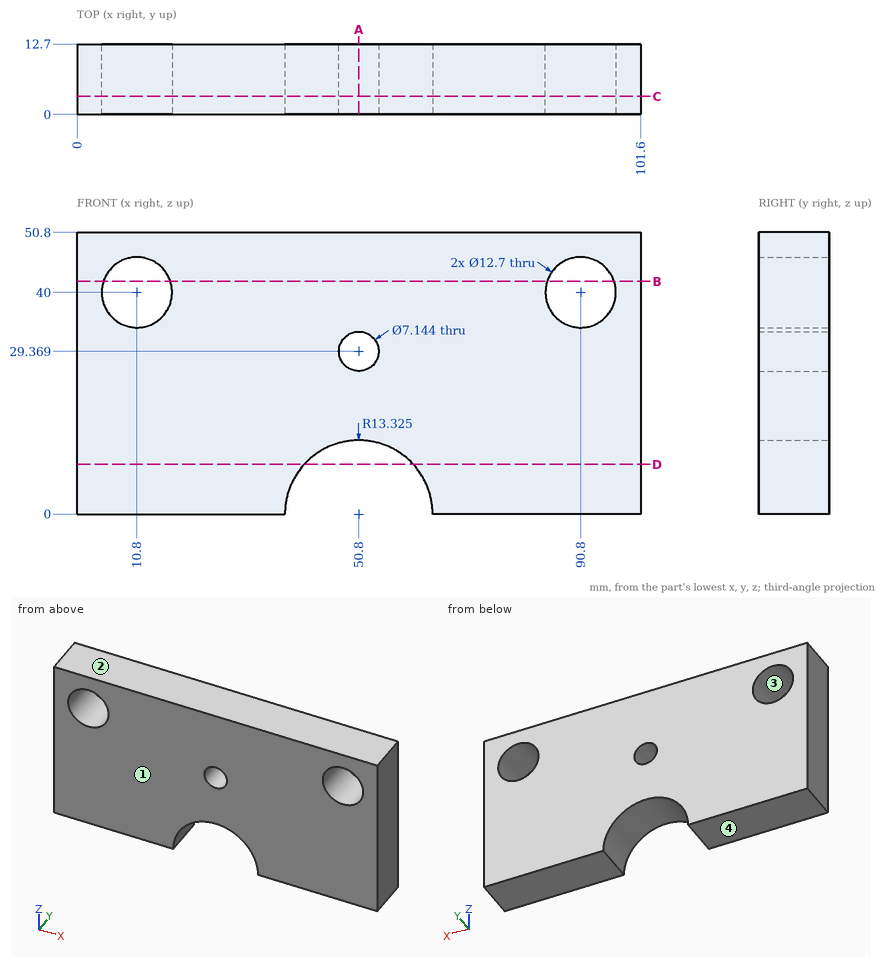
For this review, use the dimensioned drawing (mm, ordinates from the lowest corner) and the shaded views. Give positions to 0.01 mm unless a question says otherwise; leave off trailing zeros. Order: outer loops, then holes, each group sorted by start corner. A loop starts at its lowest first (then second) coordinate and runs counter-clockwise, first axis right, second up.
1. Add section A-A, the plane x = 50.8. State the section outline as (y, z) points (1 decimal).
Solution:
outline: (0, 13.3) - (12.7, 13.3) - (12.7, 25.8) - (0, 25.8) - close; (0, 32.9) - (12.7, 32.9) - (12.7, 50.8) - (0, 50.8) - close
2. To check wall thickness, follow L1, parallel to X at y = 1.25, z = 38; L2, parallel to Z at x = 10.5, y = 10.75; L3, parallel to X at y = 3, z = 44. State the ranges of each line that lie inside material, in increasing order.
Solution:
L1: x = 0 to 4.77, 16.83 to 84.77, 96.83 to 101.6
L2: z = 0 to 33.66, 46.34 to 50.8
L3: x = 0 to 5.87, 15.73 to 85.87, 95.73 to 101.6
3. Add section D-D, the plane z = 9. State the section outline as (x, y) points, then the cut area to 3 significant figures.
Solution:
outline: (0, 0) - (40.97, 0) - (40.97, 12.7) - (0, 12.7) - close; (60.63, 0) - (101.6, 0) - (101.6, 12.7) - (60.63, 12.7) - close
area: 1,040 mm2
4. Add section B-B, the plane z = 42. State the section outline as (x, y) points, then the cut area to 3 significant figures.
Solution:
outline: (0, 0) - (4.77, 0) - (4.77, 12.7) - (0, 12.7) - close; (16.83, 0) - (84.77, 0) - (84.77, 12.7) - (16.83, 12.7) - close; (96.83, 0) - (101.6, 0) - (101.6, 12.7) - (96.83, 12.7) - close
area: 984 mm2
5. Mouldability with a two-part tool opening along Z and no side actions: class the marked faces 1, 2, 3 and 4 as +Z half, -Z half, draft (parallel to the pull), parting line (faces both ways), or undercut.
Solution:
face 1: draft
face 2: +Z half
face 3: undercut
face 4: -Z half
6. Add section C-C, the plane y = 3.25. State how many separate pieces and enclosed holes the cut face has, then the cut area to 3 significant figures.
Solution:
separate pieces: 1
enclosed holes: 3
area: 4,590 mm2
